For this review, take the finished solid that the model builds, in its own axes (mm). Face numbers are marked on the shaded views. A direction names the side the tool comes from. Give positions to 0.01 mm unless a question says otherwise; leave off trailing zeros. Order: outer loops, then holes, each group sorted by start corner. A loop starts at its lowest first (then second) coordinate and runs counter-clockwise, first axis right, second up. Notation, with made-up numbers: M 14,-32 L 21,-32 A8 ccw 21,-22 Z; hole C 4,-20 d6. An arc over 180 degrees is marked long. Answer as CSV lines item,"result". Start each with the question number.
1. We need section B-B, the plane y = -33.5. Give the boundary of the cut face in (x, z).
2. Machinability: for the marked faces 4, 5, 6, 7 and 8, which of the approach directions +Z, -Z, +X, -X, +Y, -Y give a long, thin tool a straight path to every point of the face, cutting with its end or side? Answer none if there is none.
3. Mouldability with a two-part tool opening along Y and no side actions: class the marked faces 1, 2 and 3 as pulls with the +Y half, pulls with the -Y half, needs draft (parallel to the pull), parting line crosses it, or undercut.
4. Clearance check with flat-ended pins moving along their axes: P1, Ø6, axis at x = 6.5, z = -3.5, coming from the +Y side; P2, Ø0.8, axis at x = 1, z = -2.5, coming from the +Y side; P3, Ø2, axis at x = -3, z = -1, coming from the +Y side. State where each tip first meets the part, or that it passes through.
5. For line 1 along X through (y, z) = (-0.5, -1.5); line 2 along X through (y, z) = (10.5, -3.9); line 3 along Y through (x, z) = (-4, 0.5), list the stretches that pass through material, from the lowest coordinate up.
6. We need section A-A, the plane z = -3.5. Give the boundary of the cut face in (x, y), and give its area (3 significant figures).
7. We need section C-C, the plane x = 0. State how many separate pieces and enclosed holes the cut face has, and give its area (3 significant figures).
8. We need section D-D, the plane z = 3.5. Give the boundary of the cut face in (x, y).
from build123d import *
from build123d.topology import SkipClean

# Parameters (mm, degrees)
SZKIC1_R                     = 12
SZKIC1_R_2                   = 6
DODANIE_WYCI_GNI_CIE1_DEPTH  = 2
SZKIC3_W                     = 22
SZKIC3_H                     = 32
DODANIE_WYCI_GNI_CIE2_DEPTH  = 2
SZKIC4_W                     = 22
SZKIC4_H                     = 6
DODANIE_WYCI_GNI_CIE3_DEPTH  = 4
SZKIC5_R                     = 1.5
WYTNIJ_WYCI_GNI_CIE1_DEPTH   = 6
SZKIC6_W                     = 10
SZKIC6_H                     = 1
DODANIE_WYCI_GNI_CIE4_DEPTH  = 4
DODANIE_WYCI_GNI_CIE5_START  = 4
DODANIE_WYCI_GNI_CIE5_DEPTH  = 4
DODANIE_WYCI_GNI_CIE6_START  = 4
DODANIE_WYCI_GNI_CIE6_DEPTH  = 4
SZKIC12_R                    = 13
SZKIC12_R_2                  = 8.25
DODANIE_WYCI_GNI_CIE7_DEPTH  = 2
SZKIC13_R                    = 8.25
WYTNIJ_WYCI_GNI_CIE5_DEPTH   = 2
DODANIE_WYCI_GNI_CIE8_DEPTH  = 4
DODANIE_WYCI_GNI_CIE9_START  = -4
DODANIE_WYCI_GNI_CIE9_DEPTH  = 5.5
SZKIC16_W                    = 5
SZKIC16_H                    = 8.571884582
WYTNIJ_WYCI_GNI_CIE6_DEPTH   = 3
SZKIC17_R                    = 1.5
WYTNIJ_WYCI_GNI_CIE7_DEPTH   = 5.5
SZKIC18_R                    = 8.25
WYTNIJ_WYCI_GNI_CIE8_DEPTH   = 1
SZKIC19_W                    = 2
SZKIC19_H                    = 2
DODANIE_WYCI_GNI_CIE10_DEPTH = 1.5
WYTNIJ_WYCI_GNI_CIE9_START   = -3
SZKIC20_R                    = 10.5
WYTNIJ_WYCI_GNI_CIE9_DEPTH   = 3
SZKIC21_W                    = 16.5
SZKIC21_H                    = 17
WYTNIJ_WYCI_GNI_CIE10_DEPTH  = 3
SZKIC22_W                    = 22
SZKIC22_H                    = 17
DODANIE_WYCI_GNI_CIE11_DEPTH = 3
SZKIC24_R                    = 1.5
WYTNIJ_WYCI_GNI_CIE11_DEPTH  = 3
SFAZOWANIE1_SIZE             = 1
DODANIE_WYCI_GNI_CIE14_START = 1
DODANIE_WYCI_GNI_CIE14_DEPTH = 1
DODANIE_WYCI_GNI_CIE15_START = 1
DODANIE_WYCI_GNI_CIE15_DEPTH = 1
SZKIC30_W                    = 2.75
SZKIC30_H                    = 5.506367645
DODANIE_WYCI_GNI_CIE16_DEPTH = 1
DODANIE_WYCI_GNI_CIE17_START = 1
DODANIE_WYCI_GNI_CIE17_DEPTH = 1
SZKIC32_W                    = 2.75
SZKIC32_H                    = 5.07179677
DODANIE_WYCI_GNI_CIE18_DEPTH = 1
SZKIC33_W                    = 16.5
SZKIC33_H                    = 9.5
WYTNIJ_WYCI_GNI_CIE12_DEPTH  = 1
WYTNIJ_WYCI_GNI_CIE13_START  = -0.2
WYTNIJ_WYCI_GNI_CIE13_DEPTH  = 0.2


with BuildPart() as part:
    # Szkic1 → Dodanie-wyciągnięcie1 (new body)
    with BuildSketch(Plane.XY):
        Circle(SZKIC1_R)
        Circle(SZKIC1_R_2, mode=Mode.SUBTRACT)
    extrude(amount=DODANIE_WYCI_GNI_CIE1_DEPTH)

    # Szkic3 → Dodanie-wyciągnięcie2 (add)
    with BuildSketch(Plane.XY.offset(2)):
        with Locations((0, -20.5)):
            Rectangle(SZKIC3_W, SZKIC3_H)
    extrude(amount=-DODANIE_WYCI_GNI_CIE2_DEPTH)

    # Szkic4 → Dodanie-wyciągnięcie3 (add)
    with BuildSketch(Plane(origin=(0, 0, 0), x_dir=(-1, 0, 0), z_dir=(0, 0, -1))):
        with Locations((0, -33.5)):
            Rectangle(SZKIC4_W, SZKIC4_H)
    extrude(amount=DODANIE_WYCI_GNI_CIE3_DEPTH)

    # Szkic5 → Wytnij-wyciągnięcie1 (cut)
    with BuildSketch(Plane.XY.offset(2)):
        with Locations((-3.25, -33.5)):
            Circle(SZKIC5_R)
        with Locations((3.25, -33.5)):
            Circle(SZKIC5_R)
    extrude(amount=-WYTNIJ_WYCI_GNI_CIE1_DEPTH, mode=Mode.SUBTRACT)

    # Szkic6 → Dodanie-wyciągnięcie4 (add)
    with BuildSketch(Plane(origin=(0, 0, 0), x_dir=(-1, 0, 0), z_dir=(0, 0, -1))):
        with Locations((0, -11.5)):
            Rectangle(SZKIC6_W, SZKIC6_H)
    extrude(amount=DODANIE_WYCI_GNI_CIE4_DEPTH)

    # Szkic7 → Dodanie-wyciągnięcie5 (add)
    with BuildSketch(Plane(origin=(0, 0, 0), x_dir=(-1, 0, 0), z_dir=(0, 0, -1)).offset(DODANIE_WYCI_GNI_CIE5_START)):
        with BuildLine():
            Line((-5, 8.5), (-5, 5.5))
            Line((-5, 5.5), (-5, 3.31662479))
            ThreePointArc((-5, 3.31662479), (0, 6), (5, 3.31662479))
            Line((5, 3.31662479), (5, 5.5))
            Line((5, 5.5), (5, 8.5))
            Line((5, 8.5), (-5, 8.5))
        make_face()
    extrude(amount=-DODANIE_WYCI_GNI_CIE5_DEPTH)

    # Szkic9 → Dodanie-wyciągnięcie6 (add)
    with BuildSketch(Plane(origin=(0, 0, 0), x_dir=(-1, 0, 0), z_dir=(0, 0, -1)).offset(DODANIE_WYCI_GNI_CIE6_START)):
        with BuildLine():
            Line((-7, 8.5), (-7, 9.746794345))
            ThreePointArc((-7, 9.746794345), (0, 12), (7, 9.746794345))
            Line((7, 9.746794345), (7, 8.5))
            Line((7, 8.5), (7, -12))
            Line((7, -12), (5, -12))
            Line((5, -12), (5, 8.5))
            Line((5, 8.5), (-5, 8.5))
            Line((-5, 8.5), (-5, -12))
            Line((-5, -12), (-7, -12))
            Line((-7, -12), (-7, 8.5))
        make_face()
    extrude(amount=-DODANIE_WYCI_GNI_CIE6_DEPTH)

    # Szkic12 → Dodanie-wyciągnięcie7 (add)
    with BuildSketch(Plane.XY.offset(2)):
        Circle(SZKIC12_R)
        Circle(SZKIC12_R_2, mode=Mode.SUBTRACT)
    extrude(amount=-DODANIE_WYCI_GNI_CIE7_DEPTH)

    # Szkic13 → Wytnij-wyciągnięcie5 (cut)
    with BuildSketch(Plane.XY.offset(2)):
        Circle(SZKIC13_R)
    extrude(amount=-WYTNIJ_WYCI_GNI_CIE5_DEPTH, mode=Mode.SUBTRACT)

    # Szkic14 → Dodanie-wyciągnięcie8 (add)
    with BuildSketch(Plane(origin=(0, 0, 0), x_dir=(-1, 0, 0), z_dir=(0, 0, -1))):
        with BuildLine():
            Line((-7, 10.95445115), (-7, 9.746794345))
            ThreePointArc((-7, 9.746794345), (0, 12), (7, 9.746794345))
            Line((7, 9.746794345), (7, 10.95445115))
            ThreePointArc((7, 10.95445115), (0, 13), (-7, 10.95445115))
        make_face()
    extrude(amount=DODANIE_WYCI_GNI_CIE8_DEPTH)

    # Szkic15 → Dodanie-wyciągnięcie9 (add)
    with BuildSketch(Plane(origin=(0, 0, -4), x_dir=(-1, 0, 0), z_dir=(0, 0, -1)).offset(DODANIE_WYCI_GNI_CIE9_START)):
        with BuildLine():
            Line((-7, 5.5), (7, 5.5))
            Line((7, 5.5), (7, 10.95445115))
            ThreePointArc((7, 10.95445115), (0, 13), (-7, 10.95445115))
            Line((-7, 10.95445115), (-7, 5.5))
        make_face()
    extrude(amount=DODANIE_WYCI_GNI_CIE9_DEPTH)

    # Szkic16 → Wytnij-wyciągnięcie6 (cut)
    with BuildSketch(Plane.XY.offset(2)):
        with Locations((0, 10.229933778)):
            Rectangle(SZKIC16_W, SZKIC16_H)
    extrude(amount=-WYTNIJ_WYCI_GNI_CIE6_DEPTH, mode=Mode.SUBTRACT)

    # Szkic17 → Wytnij-wyciągnięcie7 (cut)
    with BuildSketch(Plane.XY):
        with Locations((0, 10.5)):
            Circle(SZKIC17_R)
    extrude(amount=-WYTNIJ_WYCI_GNI_CIE7_DEPTH, mode=Mode.SUBTRACT)

    # Szkic18 → Wytnij-wyciągnięcie8 (cut)
    with BuildSketch(Plane.XY):
        Circle(SZKIC18_R)
    extrude(amount=-WYTNIJ_WYCI_GNI_CIE8_DEPTH, mode=Mode.SUBTRACT)

    # Szkic19 → Dodanie-wyciągnięcie10 (add)
    with BuildSketch(Plane(origin=(0, 0, -4), x_dir=(-1, 0, 0), z_dir=(0, 0, -1))):
        with Locations((-6, -4)):
            Rectangle(SZKIC19_W, SZKIC19_H)
    dodanie_wyci_gni_cie10 = extrude(amount=DODANIE_WYCI_GNI_CIE10_DEPTH)

    # Lustro1: Dodanie-wyciągnięcie10 across plane
    add(dodanie_wyci_gni_cie10.mirror(Plane(origin=(0, 0, 0), x_dir=(0, 0, 1), z_dir=(1, 0, 0))))

    # Szkic20 → Wytnij-wyciągnięcie9 (cut)
    with BuildSketch(Plane.XY.offset(2).offset(WYTNIJ_WYCI_GNI_CIE9_START)):
        Circle(SZKIC20_R)
    extrude(amount=WYTNIJ_WYCI_GNI_CIE9_DEPTH, mode=Mode.SUBTRACT)

    # Szkic21 → Wytnij-wyciągnięcie10 (cut)
    with BuildSketch(Plane.XY.offset(2)):
        with Locations((0, -15)):
            Rectangle(SZKIC21_W, SZKIC21_H)
    extrude(amount=-WYTNIJ_WYCI_GNI_CIE10_DEPTH, mode=Mode.SUBTRACT)

    # Szkic22 → Dodanie-wyciągnięcie11 (add)
    with BuildSketch(Plane.XY.offset(2)):
        with Locations((0, -22.5)):
            Rectangle(SZKIC22_W, SZKIC22_H)
    extrude(amount=DODANIE_WYCI_GNI_CIE11_DEPTH)

    # Szkic24 → Wytnij-wyciągnięcie11 (cut)
    with BuildSketch(Plane.XY.offset(5)):
        with Locations((-3, -19)):
            Circle(SZKIC24_R)
        with Locations((3, -19)):
            Circle(SZKIC24_R)
    extrude(amount=-WYTNIJ_WYCI_GNI_CIE11_DEPTH, mode=Mode.SUBTRACT)

    # Sfazowanie1
    sfazowanie1_edges = [part.edges().sort_by_distance(p)[0] for p in [
        (-1.5, 10.5, -1),
    ]]
    chamfer(sfazowanie1_edges, length=SFAZOWANIE1_SIZE - 0.0001)  # a hair under: the kernel refuses the full size

    # Szkic27 → Dodanie-wyciągnięcie14 (add)
    with SkipClean():  # the faces are left unmerged after this step: merging them gives an invalid solid
        with BuildSketch(Plane(origin=(0, 0, 0), x_dir=(-1, 0, 0), z_dir=(0, 0, -1)).offset(DODANIE_WYCI_GNI_CIE14_START)):
            with BuildLine():
                Line((-7, 7.826237921), (-7, 10.95445115))
                ThreePointArc((-7, 10.95445115), (-12.977033627, 0.772397723), (-8.25, -10.046765649))
                Line((-8.25, -10.046765649), (-8.25, -6.495190528))
                ThreePointArc((-8.25, -6.495190528), (-10.460231986, 0.912987837), (-7, 7.826237921))
            make_face()
            with BuildLine():
                Line((7, 7.826237921), (7, 10.95445115))
                ThreePointArc((7, 10.95445115), (12.977033627, 0.772397723), (8.25, -10.046765649))
                Line((8.25, -10.046765649), (8.25, -6.495190528))
                ThreePointArc((8.25, -6.495190528), (10.460231986, 0.912987837), (7, 7.826237921))
            make_face()
        extrude(amount=-DODANIE_WYCI_GNI_CIE14_DEPTH)

    # Szkic29 → Dodanie-wyciągnięcie15 (add)
    with SkipClean():  # the faces are left unmerged after this step: merging them gives an invalid solid
        with BuildSketch(Plane(origin=(0, 0, -1), x_dir=(-1, 0, 0), z_dir=(0, 0, -1)).offset(DODANIE_WYCI_GNI_CIE15_START)):
            with BuildLine():
                Line((11, -6.92820323), (11, -12))
                Line((11, -12), (5, -12))
                Line((5, -12), (5, -11))
                Line((5, -11), (5, 12))
                ThreePointArc((5, 12), (12.392304845, 3.92820323), (11, -6.92820323))
            make_face()
        extrude(amount=-DODANIE_WYCI_GNI_CIE15_DEPTH)

    # Szkic30 → Dodanie-wyciągnięcie16 (add)
    with SkipClean():  # the faces are left unmerged after this step: merging them gives an invalid solid
        with BuildSketch(Plane(origin=(0, 0, 0), x_dir=(-1, 0, 0), z_dir=(0, 0, -1))):
            with Locations((9.625, -9.246816178)):
                Rectangle(SZKIC30_W, SZKIC30_H)
        extrude(amount=DODANIE_WYCI_GNI_CIE16_DEPTH)

    # Szkic31 → Dodanie-wyciągnięcie17 (add)
    with SkipClean():  # the faces are left unmerged after this step: merging them gives an invalid solid
        with BuildSketch(Plane(origin=(0, 0, -1), x_dir=(-1, 0, 0), z_dir=(0, 0, -1)).offset(DODANIE_WYCI_GNI_CIE17_START)):
            with BuildLine():
                Line((-11, -12), (-5.939283137, -12))
                Line((-5.939283137, -12), (-5.939283137, -6.495190528))
                Line((-5.939283137, -6.495190528), (-5.939283137, 11.563948972))
                ThreePointArc((-5.939283137, 11.563948972), (-12.538929442, 3.431508187), (-11, -6.92820323))
                Line((-11, -6.92820323), (-11, -12))
            make_face()
        extrude(amount=-DODANIE_WYCI_GNI_CIE17_DEPTH)

    # Szkic32 → Dodanie-wyciągnięcie18 (add)
    with SkipClean():  # the faces are left unmerged after this step: merging them gives an invalid solid
        with BuildSketch(Plane(origin=(0, 0, 0), x_dir=(-1, 0, 0), z_dir=(0, 0, -1))):
            with Locations((-9.625, -9.464101615)):
                Rectangle(SZKIC32_W, SZKIC32_H)
        extrude(amount=DODANIE_WYCI_GNI_CIE18_DEPTH)

    # Szkic33 → Wytnij-wyciągnięcie12 (cut)
    with SkipClean():  # the faces are left unmerged after this step: merging them gives an invalid solid
        with BuildSketch(Plane(origin=(0, 0, 2), x_dir=(-1, 0, 0), z_dir=(0, 0, -1))):
            with Locations((0, -18.75)):
                Rectangle(SZKIC33_W, SZKIC33_H)
        extrude(amount=-WYTNIJ_WYCI_GNI_CIE12_DEPTH, mode=Mode.SUBTRACT)

    # Wytnij-wyciągnięcie13: read off the stored shape, not the designer's step
    # Wytnij-wyciągnięcie13 outline → Wytnij-wyciągnięcie13 (cut)
    with SkipClean():  # the faces are left unmerged after this step: merging them gives an invalid solid
        with BuildSketch(Plane.XY.offset(-1).offset(WYTNIJ_WYCI_GNI_CIE13_START)):
            with BuildLine():
                Line((-8.246211251, -6.5), (-8.25, -6.5))
                Line((-8.25, -6.5), (-8.25, -12))
                Line((-8.25, -12), (8.25, -12))
                Line((8.25, -12), (8.25, -6.5))
                Line((8.25, -6.5), (8.246211251, -6.5))
                ThreePointArc((8.246211251, -6.5), (9.892290104, 3.520311988), (2.286163597, 10.248095238))
                ThreePointArc((2.286163597, 10.248095238), (0, 8.2), (-2.286163597, 10.248095238))
                ThreePointArc((-2.286163597, 10.248095238), (-9.892290104, 3.520311988), (-8.246211251, -6.5))
            make_face()
            with BuildLine():
                Line((5, 3.31662479), (5, -11))
                Line((5, -11), (-5, -11))
                Line((-5, -11), (-5, 3.31662479))
                ThreePointArc((-5, 3.31662479), (-3.856691747, 4.596295113), (-2.397915762, 5.5))
                Line((-2.397915762, 5.5), (2.397915762, 5.5))
                ThreePointArc((2.397915762, 5.5), (3.856691747, 4.596295113), (5, 3.31662479))
            make_face(mode=Mode.SUBTRACT)
        extrude(amount=WYTNIJ_WYCI_GNI_CIE13_DEPTH, mode=Mode.SUBTRACT)


solid = part.part
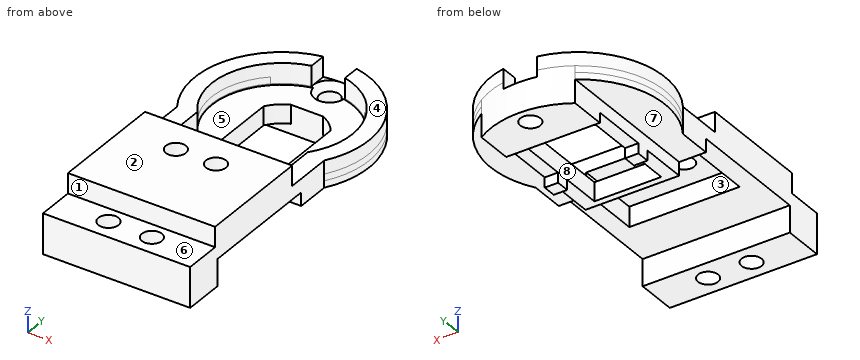
Result set:
1,outline,"M -11,-4 L -4.75,-4 L -4.75,2 L -11,2 Z; M -1.75,-4 L 1.75,-4 L 1.75,2 L -1.75,2 Z; M 4.75,-4 L 11,-4 L 11,2 L 4.75,2 Z"
2,face 4,"+Z, +X, -X, +Y"
2,face 5,"+Z"
2,face 6,"+Z, +X, -X, -Y"
2,face 7,"-Z, -X, +Y"
2,face 8,"+Z, -Z"
3,face 1,"pulls with the -Y half"
3,face 2,"needs draft"
3,face 3,"undercut"
4,P1,"y = 12.52"
4,P2,"y = 12.99"
4,P3,"y = 12.85"
5,line 1,"-12.99 to -5, 5 to 12.99"
5,line 2,"-7 to -1.5, 1.5 to 7"
5,line 3,"-36.5 to -34.8, -32.2 to -23.5, 9.71 to 12.37"
6,outline,"M -11,-36.5 L 11,-36.5 L 11,-30.5 L -11,-30.5 Z; M -7,-12 L 7,-12 L 7,10.95 A13 ccw -7,10.95 Z; hole M -5,-11 L 5,-11 L 5,3.32 A6 ccw 2.4,5.5 L -2.4,5.5 A6 ccw -5,3.32 Z; hole C -3.25,-33.5 d3; hole C 0,10.5 d3; hole C 3.25,-33.5 d3"
6,area,"291 mm2"
7,separate pieces,"4"
7,enclosed holes,"0"
7,area,"113 mm2"
8,outline,"M -11,-31 L 11,-31 L 11,-14 L -11,-14 Z; hole C -3,-19 d3; hole C 3,-19 d3"
